Study the drawing (mm; zero at the part's minimum x, y, z) and answer. Coordinates: 2 decimals unless noted, no trailing zeros. Write each loop counter-clockwise with the first axis right and the second up, starting at its lowest first coordinate (ties: lowest second). Pieces come first, ordered by that corner, then holes. Notation, with made-up numbers: M 79,-25 L 116,-25 A25 cw 116,4 Z; hole C -10,47 d2. An arc over 180 degrees is marked long. Answer as CSV lines item,"result". Start each with the question number.
(1) A cutting plane is placed at A-A on y = 56.5. Give the vertices of the cut face in (x, z), then the cut area to 3 significant figures.
(2) A flat-ended cylindrical pin translates along its axis: P1, Ø3, axis at x = 120.5, z = 3, coming from the -Y side. Find the tip coordinate at first contact, or state that the pin passes through.
(3) Find the intervals of material crossed by L1, parallel to X at y = 67.5, z = 1.45; L2, parallel to Y at x = 118, z = 1.15, in increasing order. Write a range as [from, to].
(4) A cutting plane is placed at C-C on x = 124. Give the vertices of the cut face in (y, z).
(5) A cutting plane is placed at B-B on z = 4.4. Give the vertices of the cut face in (x, y), then the cut area to 3 significant figures.
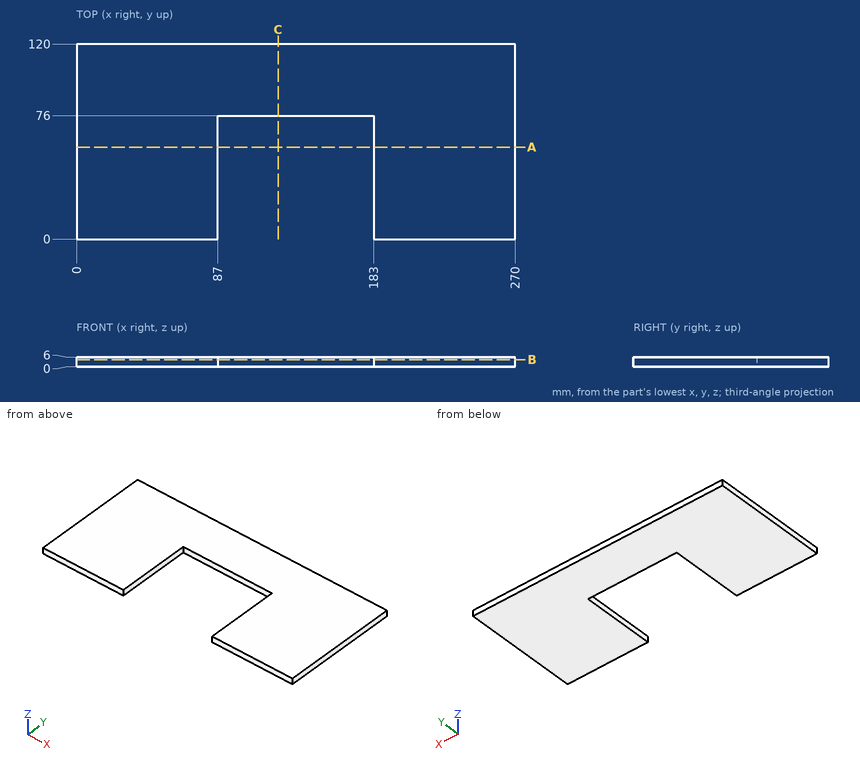
Here are the results:
1,outline,"M 0,0 L 87,0 L 87,6 L 0,6 Z; M 183,0 L 270,0 L 270,6 L 183,6 Z"
1,area,"1,040 mm^2"
2,P1,"stops at y = 76"
3,L1,"x = [0, 87], [183, 270]"
3,L2,"y = [76, 120]"
4,outline,"M 76,0 L 120,0 L 120,6 L 76,6 Z"
5,outline,"M 0,0 L 87,0 L 87,76 L 183,76 L 183,0 L 270,0 L 270,120 L 0,120 Z"
5,area,"25,100 mm^2"
